```python
from build123d import *

# Parameters (mm, degrees)
SKETCH_1_R          = 25
EXTRUDE_1_DEPTH     = 250
SKETCH_2_W          = 14
SKETCH_2_H          = 10
CUT_EXTRUDE_1_DEPTH = 100
SKETCH_3_R          = 8
CUT_EXTRUDE_2_DEPTH = 40


with BuildPart() as part:
    # 草图1 → 凸台-拉伸1 (new body)
    with BuildSketch(Plane(origin=(0, 0, 0), x_dir=(0, -1, 0), z_dir=(0, 0, 1))):
        with Locations(Location((0, 0, 0), (0, 0, 90))):
            Circle(SKETCH_1_R)
    extrude(amount=EXTRUDE_1_DEPTH)

    # 草图2 → 切除-拉伸1 (cut)
    with BuildSketch(Plane(origin=(0, 0, 250), x_dir=(0, -1, 0), z_dir=(0, 0, 1))):
        with Locations((0, 23.5)):
            Rectangle(SKETCH_2_W, SKETCH_2_H)
    extrude(amount=-CUT_EXTRUDE_1_DEPTH, mode=Mode.SUBTRACT)

    # 草图3 → 切除-拉伸2 (cut)
    with BuildSketch(Plane.XY.offset(250)):
        Circle(SKETCH_3_R)
    extrude(amount=-CUT_EXTRUDE_2_DEPTH, mode=Mode.SUBTRACT)


solid = part.part
```
Model file for the job. Use its own axes, mm. A direction names the side the tool comes from. Round coordinates to 2 decimals unless told otherwise and drop trailing zeros. Write each loop counter-clockwise with the first axis right and the second up, starting at its lowest first coordinate (ties: lowest second). Pieces come first, ordered by that corner, then holes. Notation, with made-up numbers: (-17.5, 44.25) - (29.5, 44.25) arc R10 cw to (29.5, 58.25) - close; hole circle Ø11 at (33.5, 63.25). An arc over 180 degrees is marked (long way). Use CSV: the item, a comma, the result in double quotes. Start each with the question number.
Item 1: Band-saw the part on B-B (y = 0). Write the cut outline in (x, z), and give its area (3 significant figures).
Item 2: Tool access for faces 1 (the face through (21, -7, 201)), 2 (the face through (0, 0, 210)), 3 (the face through (-6.3, -5.2, 250)): list every direction of +Z, -Z, +X, -X, +Y, -Y with a clear straight run to the whole face (end or side of a thin tool).
Item 3: Band-saw the part on D-D (z = 26). Write the cut outline in (x, y).
Item 4: Two-plate mould, pull along Y, no slides. Class faces 4 (the face through (21, 7, 201)), 5 (the face through (0, 0, 0)), 6 (the face through (23.846, 7.509, 123.25)): released by +Y, released by -Y, zero draft, split by the parting line, or undercut.
Item 5: Band-saw the part on A-A (x = 0). Write the cut outline in (y, z), and give its area (3 significant figures).
Item 6: Pin check, flat tips, straight feed: P1, Ø7, axis at y = -2, z = 218, coming from the +X side; P2, Ø4, axis at y = -11.5, z = 99.5, coming from the +X side; P3, Ø6, axis at x = -7.5, z = 55, coming from the +Y side. Stop position of each tip, or through.
Item 7: Drill centre lines: L1, parallel to Y at x = 0, z = 225; L2, parallel to X at y = -4.5, z = 190.5; L3, parallel to X at y = 10, z = 224. Where is each one in solid material? Low to high. Write a range as [from, to].
Item 8: Band-saw the part on C-C (z = 195). Write the cut outline in (x, y).
Checked values:
1,outline,"(-25, 0) - (25, 0) - (25, 150) - (18.5, 150) - (18.5, 250) - (8, 250) - (8, 210) - (-8, 210) - (-8, 250) - (-25, 250) - close"
1,area,"11,200 mm²"
2,face 1,"+Z, +X"
2,face 2,"+Z"
2,face 3,"+Z, +X, -X, +Y, -Y"
3,outline,"circle Ø50 at (0, 0)"
4,face 4,"undercut"
4,face 5,"zero draft"
4,face 6,"split by the parting line"
5,outline,"(-25, 0) - (25, 0) - (25, 250) - (8, 250) - (8, 210) - (-8, 210) - (-8, 250) - (-25, 250) - close"
5,area,"11,900 mm²"
6,P1,"stops at x = 18.5"
6,P2,"stops at x = 23.12"
6,P3,"stops at y = 24.59"
7,L1,"y = [-25, -8], [8, 25]"
7,L2,"x = [-24.59, 18.5]"
7,L3,"x = [-22.91, 22.91]"
8,outline,"(18.5, -7) - (18.5, 7) - (24, 7) arc R25 ccw (long way) to (24, -7) - close"
